Autodesk Inventor part; units mm, degrees
ref_plane "YZ Plane" through (0, 0, 0) normal (1, 0, 0) x (0, 1, 0)
ref_plane "XZ Plane" through (0, 0, 0) normal (0, 1, 0) x (-1, 0, 0)
ref_plane "XY Plane" through (0, 0, 0) normal (0, 0, 1) x (1, 0, 0)
sketch "Sketch5" plane through (0, 0, 0) normal (0, 0, 1) x (1, 0, 0)
  line L0 (0, 0) -> (6.35, 0)
  line L1 (6.35, 0) -> (6.35, 25.4)
  line L2 (6.35, 25.4) -> (0, 25.4)
  line L3 (0, 25.4) -> (0, 0)
  dimension "d21" = 25.4
  dimension "d22" = 6.35
extrude "Extrusion3" add sketch "Sketch5" against normal mid plane 38.1
sketch "Sketch6" plane through (0, 0, 0) normal (0, 0, 1) x (1, 0, 0)
  line L0 (6.35, 25.4) -> (6.35, 0)
  line L1 (0, 25.4) -> (6.35, 25.4)
  line L2 (6.35, 0) -> (0, 0)
  line L3 (0, 0) -> (0, 25.4)
  line L4 (6.35, 0) -> (108.9025, 37.3261)
  line L5 (6.35, 0) -> (115.4841, 0) construction
  line L6 (108.9025, 62.7261) -> (108.9025, 37.3261)
  arc A0 (76.0708, 50.7763) -> (101.7292, 60.1152) centre (88.9, 55.4457) ccw
  line L7 (6.35, 25.4) -> (76.0708, 50.7763)
  line L8 (101.7292, 60.1152) -> (108.9025, 62.7261)
  dimension "d25" = 20
  dimension "d26" = 27.305
  dimension "d29" = 6.35
  dimension "d30" = 88.9
  dimension "d33" = 0
extrude "Extrusion4" add sketch "Sketch6" along normal mid plane 6.35 contours L7 A0 L8 L6 L4 L0
sketch "Sketch7" plane through (6.35, 0, 19.05) normal (1, 0, 0) x (0, 0, -1)
  line L0 (38.1, 25.4) -> (0, 25.4) construction
  line L1 (6.35, 25.4) -> (6.35, 0) construction
  line L2 (31.75, 25.4) -> (31.75, 0) construction
  line L3 (0, 0) -> (0, 25.4) construction
  line L4 (38.1, 25.4) -> (38.1, 0) construction
  line L5 (0, 0) -> (15.875, 0)
  line L6 (22.225, 0) -> (38.1, 0)
  point P0 (19.05, 0)
  point P1 (6.35, 12.7)
  point P2 (31.75, 12.7)
  dimension "d34" = 6.35
  dimension "d35" = 6.35
sketch "Sketch8" plane through (0, 0, 0) normal (0, 0, 1) x (1, 0, 0)
  line L0 (0, 0) -> (0, 25.4)
  line L1 (6.35, 0) -> (0, 0)
  line L2 (108.9025, 37.3261) -> (6.35, 0)
  line L3 (0, 0) -> (6.35, 0)
  line L4 (0, -2.3112) -> (6.35, 0)
  line L5 (0, 0) -> (0, -2.3112)
extrude "Extrusion5" add sketch "Sketch8" along normal mid plane 38.1
hole "Hole3" at (6.35, 12.7, 12.7) at (6.35, 12.7, -12.7) direction (-1, 0, 0) diameter 3.81 end through all countersink diameter 7.0866 countersink angle 82
equation "\"d21\" = supportHeight"
equation "\"d22\" = supportWidth"
equation "\"d23\" = totalScrewHoldWidth"
equation "\"d25\" = supportAngle"
equation "\"d26\" = pipeDiameter"
equation "\"d30\" = distanceFromWallToPipeCenter"
equation "\"d31\" = supportWidth"
equation "\"d47\" = totalScrewHoldWidth"
equation "\"pipeDiameter\" = 27.305"
equation "\"distanceFromWallToPipeCenter\" = 88.9"
equation "\"supportHeight\" = 25.4"
equation "\"supportWidth\" = 6.35"
equation "\"screwHoldDepth\" = 6.35"
equation "\"totalScrewHoldWidth\" = 38.1"
equation "\"screwPositionFromTop\" = 6.35"
equation "\"supportAngle\" = 20deg"
properties part number "PipeSupport-3_50-020"
Verification items for the finished model (mm, model axes). A direction names the side the tool comes from. Round coordinates to 2 decimals unless told otherwise and drop trailing zeros. Loops run counter-clockwise (first coordinate to the right, second up) from the corner with the lowest first, then second, coordinate; pieces in that order, holes last. Notation, with made-up numbers: (22, 54.25) - (63, 54.25) arc R15 cw to (63, 80.25) - close; hole circle Ø3 at (50.5, 50). An arc over 180 degrees is marked (long way). Write item = value, one per line.
Q1. Sectioned sample at B-B on y = 44. Record the boundary of the cut face in (x, z) (1 decimal), plus the area to 3 significant figures.
Here are the results:
outline = (57.5, -3.2) - (81.5, -3.2) - (81.5, 3.2) - (57.5, 3.2) - close; (96.3, -3.2) - (108.9, -3.2) - (108.9, 3.2) - (96.3, 3.2) - close
area = 232 mm^2
Q2. Depth check by flat-ended pin: pin 1 (19 mm diameter, centred on x = 79.5, y = 17.5, fed in from -Z) (3 decimals); pin 2 (1.9 mm diameter, centred on x = 2.5, z = -2, fed in from +Y); pin 3 (8 mm diameter, centred on y = 16, z = -11.5, fed in from +X); pin 4 (3.5 mm diameter, centred on y = 12.7, z = 12.7, fed in from +X). Enter the tip coordinate at first touch or a pass-through.
Here are the results:
pin_1 = -3.175
pin_2 = 25.4
pin_3 = 6.35
pin_4 = through
Q3. Sectioned sample at A-A on z = 12.7. Record the boundary of the cut face in (x, y) (3 decimals).
Here are the results:
outline = (0, -2.311) - (6.35, 0) - (6.35, 9.157) - (4.465, 10.795) - (0, 10.795) - close; (0, 14.605) - (4.465, 14.605) - (6.35, 16.243) - (6.35, 25.4) - (0, 25.4) - close
Q4. Material ranges on L1, parallel to Z at x = 1.5, y = 12.7 (3 decimals); L2, parallel to Z at x = 3, y = 12; L3, parallel to Z at x = 78, y = 31 (3 decimals), recorded low to high.
Here are the results:
L1 = -19.05 to -14.605, -10.795 to 10.795, 14.605 to 19.05
L2 = -19.05 to -14.47, -10.93 to 10.93, 14.47 to 19.05
L3 = -3.175 to 3.175
Q5. Sectioned sample at C-C on y = 12.7. Record the boundary of the cut face in (x, z) (3 decimals).
Here are the results:
outline = (0, -19.05) - (6.35, -19.05) - (6.35, -16.243) - (4.465, -14.605) - (0, -14.605) - close; (0, -10.795) - (4.465, -10.795) - (6.35, -9.157) - (6.35, -3.175) - (41.243, -3.175) - (41.243, 3.175) - (6.35, 3.175) - (6.35, 9.157) - (4.465, 10.795) - (0, 10.795) - close; (0, 14.605) - (4.465, 14.605) - (6.35, 16.243) - (6.35, 19.05) - (0, 19.05) - close
Q6. Mould release check, pull along Y, two halves, no side actions. Record for faces 1 (the flat face through (6.35, 15, -9)), 2 (the cylindrical face through (93.85, 42.72, -0.04)), 3 (the flat face through (40.72, 37.91, -0.04)): +Y half, -Y half, draft (parallel to the pull), parting line (faces both ways), or undercut.
Here are the results:
face_1 = draft
face_2 = undercut
face_3 = +Y half
Q7. Tool access check on faces 4 (the conical face through (4.583, 14.057, -11.22)), 5 (the flat face through (6.35, 10, 9)), 6 (the flat face through (57, 32, -3.175)). Record the directions out of +Z, -Z, +X, -X, +Y, -Y that give a thin tool (end or side, any length) a straight path to the whole face; none if there is none.
Here are the results:
face_4 = +X
face_5 = +Z, +X, +Y, -Y
face_6 = -Z, +X, +Y, -Y
Q8. Sectioned sample at D-D on z = -6. Record the boundary of the cut face in (x, y).
Here are the results:
outline = (0, -2.31) - (6.35, 0) - (6.35, 25.4) - (0, 25.4) - close
